Autodesk Inventor part; units mm, degrees
ref_plane "YZ Plane" through (0, 0, 0) normal (1, 0, 0) x (0, 1, 0)
ref_plane "XZ Plane" through (0, 0, 0) normal (0, 1, 0) x (-1, 0, 0)
ref_plane "XY Plane" through (0, 0, 0) normal (0, 0, 1) x (1, 0, 0)
sketch "Sketch1" plane through (0, 0, 0) normal (0, 0, 1) x (1, 0, 0)
  line L0 (0, 3) -> (-4, 3)
  line L1 (0, 0) -> (0, 4)
  line L2 (8.5, 4) -> (0, 4)
  line L3 (8.5, 4) -> (8.5, 0)
  line L4 (13.5, 0) -> (8.5, 0)
  line L5 (13.5, 0) -> (13.5, 4)
  line L6 (18.5, 4) -> (13.5, 4)
  line L7 (18.5, 4) -> (18.5, 0)
  line L8 (23.5, 0) -> (18.5, 0)
  line L9 (23.5, 0) -> (23.5, 4)
  line L10 (28.5, 4) -> (23.5, 4)
  line L11 (28.5, 4) -> (28.5, 0)
  line L12 (33.5, 0) -> (28.5, 0)
  line L13 (33.5, 0) -> (33.5, 4)
  line L14 (38.5, 4) -> (33.5, 4)
  line L15 (38.5, 4) -> (38.5, 0)
  line L16 (43.5, 0) -> (38.5, 0)
  line L17 (43.5, 0) -> (43.5, 4)
  line L18 (48.5, 4) -> (43.5, 4)
  line L19 (48.5, 4) -> (48.5, 0)
  line L20 (53.5, 0) -> (48.5, 0)
  line L21 (53.5, 0) -> (53.5, 4)
  line L22 (58.5, 4) -> (53.5, 4)
  line L23 (58.5, 4) -> (58.5, 0)
  line L24 (63.5, 0) -> (58.5, 0)
  line L25 (63.5, 0) -> (63.5, 4)
  line L26 (68.5, 4) -> (63.5, 4)
  line L27 (68.5, 4) -> (68.5, 0)
  line L28 (73.5, 0) -> (68.5, 0)
  line L29 (73.5, 0) -> (73.5, 4)
  line L30 (78.5, 4) -> (73.5, 4)
  line L31 (83.5, 0) -> (78.5, 0)
  line L32 (78.5, 4) -> (78.5, 0)
  line L33 (83.5, 0) -> (83.5, 4)
  line L34 (88.5, 4) -> (83.5, 4)
  line L35 (88.5, 4) -> (88.5, 0)
  line L36 (93.5, 0) -> (88.5, 0)
  line L37 (93.5, 0) -> (93.5, 4)
  line L38 (98.5, 4) -> (93.5, 4)
  line L39 (98.5, 4) -> (98.5, 0)
  line L40 (103.5, 0) -> (98.5, 0)
  line L41 (103.5, 0) -> (103.5, 4)
  line L42 (108.5, 4) -> (103.5, 4)
  line L43 (108.5, 4) -> (108.5, 0)
  line L44 (113.5, 0) -> (108.5, 0)
  line L45 (113.5, 0) -> (113.5, 4)
  line L46 (122, 4) -> (113.5, 4)
  line L47 (126, 3) -> (122, 3)
  line L48 (122, 0) -> (122, 4)
  line L49 (126, 8) -> (126, 3)
  line L50 (126, 8) -> (122, 8)
  line L51 (122, 8) -> (122, 13)
  line L52 (126, 13) -> (122, 13)
  line L53 (126, 18) -> (126, 13)
  line L54 (126, 18) -> (122, 18)
  line L55 (122, 18) -> (122, 23)
  line L56 (126, 23) -> (122, 23)
  line L57 (126, 28) -> (126, 23)
  line L58 (126, 28) -> (122, 28)
  line L59 (122, 28) -> (122, 33)
  line L60 (126, 33) -> (122, 33)
  line L61 (126, 38) -> (126, 33)
  line L62 (126, 38) -> (122, 38)
  line L63 (122, 38) -> (122, 43)
  line L64 (126, 43) -> (122, 43)
  line L65 (126, 48) -> (126, 43)
  line L66 (126, 48) -> (122, 48)
  line L67 (122, 48) -> (122, 53)
  line L68 (126, 53) -> (122, 53)
  line L69 (126, 58) -> (126, 53)
  line L70 (126, 58) -> (122, 58)
  line L71 (122, 58) -> (122, 68)
  line L72 (-4, 8) -> (-4, 3)
  line L73 (0, 8) -> (-4, 8)
  line L74 (0, 13) -> (0, 8)
  line L75 (0, 13) -> (-4, 13)
  line L76 (-4, 18) -> (-4, 13)
  line L77 (0, 18) -> (-4, 18)
  line L78 (0, 23) -> (0, 18)
  line L79 (0, 23) -> (-4, 23)
  line L80 (-4, 28) -> (-4, 23)
  line L81 (0, 28) -> (-4, 28)
  line L82 (0, 33) -> (0, 28)
  line L83 (-4, 33) -> (0, 33)
  line L84 (-4, 38) -> (-4, 33)
  line L85 (0, 38) -> (-4, 38)
  line L86 (0, 43) -> (0, 38)
  line L87 (0, 43) -> (-4, 43)
  line L88 (-4, 48) -> (-4, 43)
  line L89 (0, 48) -> (-4, 48)
  line L90 (0, 53) -> (0, 48)
  line L91 (-4, 53) -> (0, 53)
  line L92 (-4, 58) -> (-4, 53)
  line L93 (0, 58) -> (-4, 58)
  line L94 (0, 68) -> (0, 58)
  line L95 (0, 64) -> (122, 64)
  point P0 (0, 0)
extrude "Extrusion1" add sketch "Sketch1" along normal blind 4
sketch "Sketch2" plane through (0, 0, 0) normal (0, 0, -1) x (-1, 0, 0)
  line L0 (-8.5, 4) -> (-8.5, 0)
  line L1 (0, 4) -> (-8.5, 4)
  line L2 (0, 3) -> (0, 4)
  line L3 (4, 3) -> (0, 3)
  line L4 (4, 8) -> (4, 3)
  line L5 (0, 8) -> (4, 8)
  line L6 (0, 13) -> (0, 8)
  line L7 (4, 13) -> (0, 13)
  line L8 (4, 18) -> (4, 13)
  line L9 (0, 18) -> (4, 18)
  line L10 (0, 23) -> (0, 18)
  line L11 (4, 23) -> (0, 23)
  line L12 (4, 28) -> (4, 23)
  line L13 (0, 28) -> (4, 28)
  line L14 (0, 33) -> (0, 28)
  line L15 (4, 33) -> (0, 33)
  line L16 (4, 38) -> (4, 33)
  line L17 (0, 38) -> (4, 38)
  line L18 (0, 43) -> (0, 38)
  line L19 (4, 43) -> (0, 43)
  line L20 (4, 48) -> (4, 43)
  line L21 (0, 48) -> (4, 48)
  line L22 (0, 53) -> (0, 48)
  line L23 (4, 53) -> (0, 53)
  line L24 (4, 58) -> (4, 53)
  line L25 (0, 58) -> (4, 58)
  line L26 (0, 64) -> (0, 58)
  line L27 (-122, 64) -> (0, 64)
  line L28 (-122, 58) -> (-122, 64)
  line L29 (-126, 58) -> (-122, 58)
  line L30 (-126, 53) -> (-126, 58)
  line L31 (-122, 53) -> (-126, 53)
  line L32 (-122, 48) -> (-122, 53)
  line L33 (-126, 48) -> (-122, 48)
  line L34 (-126, 43) -> (-126, 48)
  line L35 (-122, 43) -> (-126, 43)
  line L36 (-122, 38) -> (-122, 43)
  line L37 (-126, 38) -> (-122, 38)
  line L38 (-126, 33) -> (-126, 38)
  line L39 (-122, 33) -> (-126, 33)
  line L40 (-122, 28) -> (-122, 33)
  line L41 (-126, 28) -> (-122, 28)
  line L42 (-126, 23) -> (-126, 28)
  line L43 (-122, 23) -> (-126, 23)
  line L44 (-122, 18) -> (-122, 23)
  line L45 (-126, 18) -> (-122, 18)
  line L46 (-126, 13) -> (-126, 18)
  line L47 (-122, 13) -> (-126, 13)
  line L48 (-122, 8) -> (-122, 13)
  line L49 (-126, 8) -> (-122, 8)
  line L50 (-126, 3) -> (-126, 8)
  line L51 (-122, 3) -> (-126, 3)
  line L52 (-122, 4) -> (-122, 3)
  line L53 (-113.5, 4) -> (-122, 4)
  line L54 (-113.5, 0) -> (-113.5, 4)
  line L55 (-108.5, 0) -> (-113.5, 0)
  line L56 (-108.5, 4) -> (-108.5, 0)
  line L57 (-103.5, 4) -> (-108.5, 4)
  line L58 (-103.5, 0) -> (-103.5, 4)
  line L59 (-98.5, 0) -> (-103.5, 0)
  line L60 (-98.5, 4) -> (-98.5, 0)
  line L61 (-93.5, 4) -> (-98.5, 4)
  line L62 (-93.5, 0) -> (-93.5, 4)
  line L63 (-88.5, 0) -> (-93.5, 0)
  line L64 (-88.5, 4) -> (-88.5, 0)
  line L65 (-83.5, 4) -> (-88.5, 4)
  line L66 (-83.5, 0) -> (-83.5, 4)
  line L67 (-78.5, 0) -> (-83.5, 0)
  line L68 (-78.5, 4) -> (-78.5, 0)
  line L69 (-73.5, 4) -> (-78.5, 4)
  line L70 (-73.5, 0) -> (-73.5, 4)
  line L71 (-68.5, 0) -> (-73.5, 0)
  line L72 (-68.5, 4) -> (-68.5, 0)
  line L73 (-63.5, 4) -> (-68.5, 4)
  line L74 (-63.5, 0) -> (-63.5, 4)
  line L75 (-58.5, 0) -> (-63.5, 0)
  line L76 (-58.5, 4) -> (-58.5, 0)
  line L77 (-53.5, 4) -> (-58.5, 4)
  line L78 (-53.5, 0) -> (-53.5, 4)
  line L79 (-48.5, 0) -> (-53.5, 0)
  line L80 (-48.5, 4) -> (-48.5, 0)
  line L81 (-43.5, 4) -> (-48.5, 4)
  line L82 (-43.5, 0) -> (-43.5, 4)
  line L83 (-38.5, 0) -> (-43.5, 0)
  line L84 (-38.5, 4) -> (-38.5, 0)
  line L85 (-33.5, 4) -> (-38.5, 4)
  line L86 (-33.5, 0) -> (-33.5, 4)
  line L87 (-28.5, 0) -> (-33.5, 0)
  line L88 (-28.5, 4) -> (-28.5, 0)
  line L89 (-23.5, 4) -> (-28.5, 4)
  line L90 (-23.5, 0) -> (-23.5, 4)
  line L91 (-18.5, 0) -> (-23.5, 0)
  line L92 (-18.5, 4) -> (-18.5, 0)
  line L93 (-13.5, 4) -> (-18.5, 4)
  line L94 (-13.5, 0) -> (-13.5, 4)
  line L95 (-8.5, 0) -> (-13.5, 0)
  point P0 (0, 0)
properties part number "BackWand"
Geometry check sheet. Reference: the model listing, model coordinates, mm. A direction names the side the tool comes from. Round coordinates to 2 decimals unless told otherwise and drop trailing zeros. Order: outer loops, then holes, each group sorted by start corner. A loop starts at its lowest first (then second) coordinate and runs counter-clockwise, first axis right, second up. Notation, with made-up numbers: (-30.5, 33) -> (26.5, 33) arc R19 cw to (26.5, 41) -> close; hole circle Ø3 at (-12.5, 24). An arc over 180 degrees is marked (long way). Use one line per item in the form item = value.
1. Cross-section at A-A, the plane y = 19.5. Enter the section's corners in (x, z), plus the area to 3 significant figures.
Working result:
outline = (0, 0) -> (122, 0) -> (122, 4) -> (0, 4) -> close
area = 488 mm^2
2. Go/stop test with flat-tipped pins: pin 1 (2 mm diameter, centred on x = -2, z = 1.5, fed in from +Y); pin 2 (1.5 mm diameter, centred on x = 67, z = 2, fed in from -Y); pin 3 (4 mm diameter, centred on x = 38, y = 49, fed in from -Z). Record where each tip stops, or that it passes through.
Working result:
pin_1 = 58
pin_2 = 4
pin_3 = 0
3. Set-up check for faces 1 (the face through (126, 36, 2)), 2 (the face through (124, 53, 2)), 3 (the face through (0, 31, 2)), 4 (the face through (11, 0, 2)), 5 (the face through (13.5, 2, 2)): record each of +Z, -Z, +X, -X, +Y, -Y from which the full face is reachable in a straight line by a thin tool's end or side.
Working result:
face_1 = +Z, -Z, +X, +Y, -Y
face_2 = +Z, -Z, +X
face_3 = +Z, -Z, -X
face_4 = +Z, -Z, +X, -X, -Y
face_5 = +Z, -Z, -Y
4. Scan lines: line 1 along X through (y, z) = (29.5, 3.1); line 2 along Y through (x, z) = (107, 0.75). Record each from-to range of solid material in increasing order. Write a range as from..to.
Working result:
line_1 = 0..122
line_2 = 4..64
5. Mould release check, pull along Y, two halves, no side actions. Record for faces 6 (the face through (-2, 33, 2)), 7 (the face through (108.5, 2, 2)), 8 (the face through (16, 4, 2)): pulls with the +Y half, pulls with the -Y half, needs draft (parallel to the pull), parting line crosses it, or undercut.
Working result:
face_6 = undercut
face_7 = needs draft
face_8 = pulls with the -Y half
